Source: three-view drawing plus pictorial views. Frame: mm from the lowest corner of the part. Round coordinates to 2 decimals unless told otherwise and drop trailing zeros. Loops run counter-clockwise (first coordinate to the right, second up) from the corner with the lowest first, then second, coordinate; pieces in that order, holes last. Notation, with made-up numbers: M 48,7.5 L 93,7.5 A30 ccw 93,46.5 Z; hole C 11.25,-8.5 d11. An arc over 180 degrees is marked long. Return JSON: item names as keys, results as strings. Group by question number.
1) Section B-B (x = 9.9). Output: boundary loops of the cut face in (y, z), plus the area to 3 significant figures.
2) Material intervals for line 1 (X direction, y = 0.5, z = 3.4); line 2 (Z direction, x = 3.5, y = 0.15); line 3 (Z direction, x = 18.75, y = 0.5), sorted ascending. Write a range as from..to.
3) Section A-A (z = 15.75). Output: boundary loops of the cut face in (x, y), plus the area to 3 significant figures.
4) Section D-D (x = 3.9). Output: boundary loops of the cut face in (y, z), plus the area to 3 significant figures.
5) Contact query for a flat-ended pin moving along its axis: P1, Ø3, axis at x = 3.9, z = 3.4, coming from the +Y side. Output: stop coordinate, or through.
6) Section C-C (y = 0.85). Output: boundary loops of the cut face in (x, z).
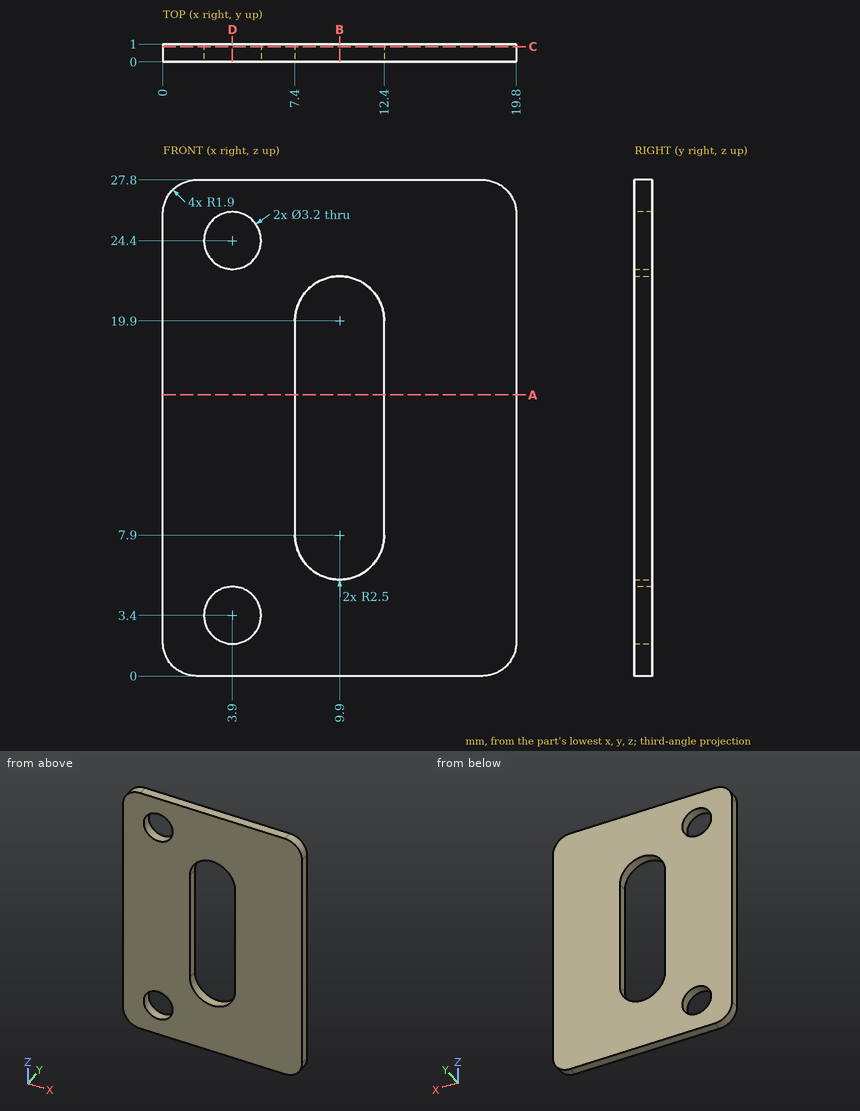
Returned:
{
 "1": {"outline": "M 0,0 L 1,0 L 1,5.4 L 0,5.4 Z; M 0,22.4 L 1,22.4 L 1,27.8 L 0,27.8 Z", "area": "10.8 mm^2"},
 "2": {"line 1": "x = 0..2.3, 5.5..19.8", "line 2": "z = 0..1.85, 4.95..22.85, 25.95..27.8", "line 3": "z = 0.2..27.6"},
 "3": {"outline": "M 0,0 L 7.4,0 L 7.4,1 L 0,1 Z; M 12.4,0 L 19.8,0 L 19.8,1 L 12.4,1 Z", "area": "14.8 mm^2"},
 "4": {"outline": "M 0,0 L 1,0 L 1,1.8 L 0,1.8 Z; M 0,5 L 1,5 L 1,22.8 L 0,22.8 Z; M 0,26 L 1,26 L 1,27.8 L 0,27.8 Z", "area": "21.4 mm^2"},
 "5": {"P1": "passes through"},
 "6": {"outline": "M 0,1.9 A1.9 ccw 1.9,0 L 17.9,0 A1.9 ccw 19.8,1.9 L 19.8,25.9 A1.9 ccw 17.9,27.8 L 1.9,27.8 A1.9 ccw 0,25.9 Z; hole C 3.9,3.4 d3.2; hole C 3.9,24.4 d3.2; hole M 7.4,7.9 A2.5 ccw 12.4,7.9 L 12.4,19.9 A2.5 ccw 7.4,19.9 Z"}
}
